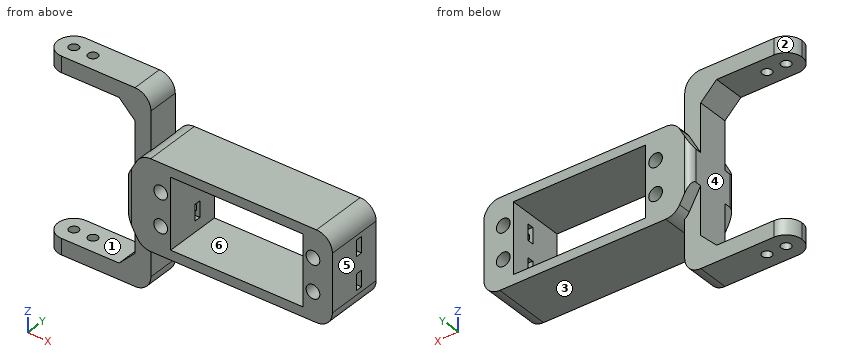
```python
from build123d import *

# Parameters (mm, degrees)
ESQUISSE1_W                         = 60
ESQUISSE1_H                         = 18
BOSS_EXTRU_1_DEPTH                  = 28
ESQUISSE2_W                         = 41.5
ESQUISSE2_H                         = 22
ENL_V_MAT_EXTRU_1_DEPTH             = 30
ESQUISSE3_R                         = 2.15
ENL_V_MAT_EXTRU_2_DEPTH             = 30
ESQUISSE5_W                         = 10
ESQUISSE5_H                         = 60
BOSS_EXTRU_2_DEPTH                  = 5
ESQUISSE6_W                         = 10
ESQUISSE6_H                         = 5
BOSS_EXTRU_3_DEPTH                  = 28
ESQUISSE7_R                         = 1.5
ENL_V_MAT_EXTRU_4_DEPTH             = 92.394748208
NERVURE11_REACH                     = 77.186
ESQUISSE8_WALL_W                    = 162.668500034
ESQUISSE8_WALL_H                    = 18
CONG_5_R                            = 5
CONG_6_R                            = 5
NERVURE12_REACH                     = 73.169
ESQUISSE10_WALL_W                   = 151.408694602
ESQUISSE10_WALL_H                   = 10
CONG_7_R                            = 5
ESQUISSE12_W                        = 5
ESQUISSE12_H                        = 2
ENL_V_MAT_EXTRU_5_DEPTH             = 8
ENL_V_MAT_EXTRU_5_DIRECTION_2_REACH = 67.265
R_P_TITION_CIRCULAIRE1_COUNT        = 3
R_P_TITION_CIRCULAIRE1_ANGLE        = 180
ENL_V_MAT_EXTRU_8_DEPTH             = 79.064076245
ENL_V_MAT_EXTRU_8_DEPTH_BACK        = 79.064076245
CONG_8_R                            = 5
CONG_10_R                           = 5
CONG_12_R                           = 2
NERVURE13_REACH                     = 79.369
ESQUISSE22_WALL_W                   = 163.809556882
ESQUISSE22_WALL_H                   = 10
ENL_V_MAT_EXTRU_10_DEPTH            = 88.464278423
ENL_V_MAT_EXTRU_10_DEPTH_BACK       = 88.464278423
ESQUISSE24_R                        = 1.5


with BuildPart() as part:
    # Esquisse1 → Boss.-Extru.1 (new body)
    with BuildSketch(Plane.XY):
        Rectangle(ESQUISSE1_W, ESQUISSE1_H)
    extrude(amount=BOSS_EXTRU_1_DEPTH)

    # Esquisse2 → Enlèv. mat.-Extru.1 (cut)
    with BuildSketch(Plane.XZ.offset(9)):
        with Locations((0, 14)):
            Rectangle(ESQUISSE2_W, ESQUISSE2_H)
    extrude(amount=-ENL_V_MAT_EXTRU_1_DEPTH, mode=Mode.SUBTRACT)

    # Esquisse3 → Enlèv. mat.-Extru.2 (cut)
    with BuildSketch(Plane(origin=(0, -9, 0), x_dir=(-1, 0, 0), z_dir=(0, -1, 0))):
        with Locations(Location((23.9, -19.1, 0), (0, 0, 90))):
            Circle(ESQUISSE3_R)
        with Locations(Location((23.9, -8.9, 0), (0, 0, 90))):
            Circle(ESQUISSE3_R)
        with Locations(Location((-23.9, -8.9, 0), (0, 0, 90))):
            Circle(ESQUISSE3_R)
        with Locations(Location((-23.9, -19.1, 0), (0, 0, 90))):
            Circle(ESQUISSE3_R)
    extrude(amount=-ENL_V_MAT_EXTRU_2_DEPTH, mode=Mode.SUBTRACT)

    # Esquisse5 → Boss.-Extru.2 (add)
    with BuildSketch(Plane.ZY.offset(30)):
        with Locations((14, 0)):
            Rectangle(ESQUISSE5_W, ESQUISSE5_H)
    boss_extru_2 = extrude(amount=BOSS_EXTRU_2_DEPTH)

    # Esquisse6 → Boss.-Extru.3 (add)
    with BuildSketch(Plane.ZY.offset(35)):
        with Locations((14, 27.5)):
            Rectangle(ESQUISSE6_W, ESQUISSE6_H)
        with Locations((14, -27.5)):
            Rectangle(ESQUISSE6_W, ESQUISSE6_H)
    boss_extru_3 = extrude(amount=BOSS_EXTRU_3_DEPTH)

    # Esquisse7 → Enlèv. mat.-Extru.4 (cut, symmetric)
    with BuildSketch(Plane(origin=(0, 30, 0), x_dir=(1, 0, 0), z_dir=(0, 1, 0))):
        with Locations(Location((-58, -14, 0), (0, 0, 270))):
            Circle(ESQUISSE7_R)
    enl_v_mat_extru_4 = extrude(amount=ENL_V_MAT_EXTRU_4_DEPTH, both=True, mode=Mode.SUBTRACT)

    # Esquisse8 wall → Nervure11 (add, up to next)
    with BuildSketch(Plane(origin=(-32.5, 0, 23.5), x_dir=(-0.485642931179, 0, -0.874157276122), z_dir=(-0.874157276122, 0, 0.485642931179)), mode=Mode.PRIVATE) as nervure11_sk1:
        Rectangle(ESQUISSE8_WALL_W, ESQUISSE8_WALL_H)
    nervure11_tool1 = extrude(nervure11_sk1.sketch, amount=-NERVURE11_REACH, mode=Mode.PRIVATE) - part.part
    nervure11 = nervure11_tool1.solids().sort_by_distance((-32.5, 0, 23.5))[0]
    add(nervure11)

    # Symétrie1: Nervure11 across plane
    add(nervure11.mirror(Plane.XY.offset(14)))

    # Congé5
    cong_5_edges = [part.edges().sort_by_distance(p)[0] for p in [
        (-30, 0, 28),
        (30, 0, 28),
        (-30, 0, 0),
        (30, 0, 0),
    ]]
    fillet(cong_5_edges, radius=CONG_5_R)

    # Congé6
    cong_6_edges = [part.edges().sort_by_distance(p)[0] for p in [
        (-30, 30, 14),
        (-30, -30, 14),
    ]]
    fillet(cong_6_edges, radius=CONG_6_R)

    # Esquisse10 wall → Nervure12 (add, up to next)
    with BuildSketch(Plane(origin=(-37.5, 22.5, 14), x_dir=(0.707106781187, -0.707106781187, 0), z_dir=(0.707106781187, 0.707106781187, 0)), mode=Mode.PRIVATE) as nervure12_sk1:
        Rectangle(ESQUISSE10_WALL_W, ESQUISSE10_WALL_H)
    nervure12_tool1 = extrude(nervure12_sk1.sketch, amount=NERVURE12_REACH, mode=Mode.PRIVATE) - part.part
    nervure12 = nervure12_tool1.solids().sort_by_distance((-37.5, 22.5, 14))[0]
    add(nervure12)

    # Symétrie2: Nervure12 across plane
    add(nervure12.mirror(Plane.ZX))

    # Congé7
    cong_7_edges = [part.edges().sort_by_distance(p)[0] for p in [
        (-63, -27.5, 9),
        (-63, -27.5, 19),
        (-63, 27.5, 9),
        (-63, 27.5, 19),
    ]]
    fillet(cong_7_edges, radius=CONG_7_R - 0.0001)  # a hair under: the kernel refuses the full size

    # Esquisse12 → Enlèv. mat.-Extru.5 (cut)
    with BuildSketch(Plane(origin=(-20.75, 0, 0), x_dir=(0, 0, -1), z_dir=(1, 0, 0))):
        with Locations((-19.1, 2)):
            Rectangle(ESQUISSE12_W, ESQUISSE12_H)
        with Locations((-8.9, 2)):
            Rectangle(ESQUISSE12_W, ESQUISSE12_H)
    extrude(amount=-ENL_V_MAT_EXTRU_5_DEPTH, mode=Mode.SUBTRACT)

    # Esquisse12 → Enlèv. mat.-Extru.5 direction 2 (cut, up to next)
    with BuildSketch(Plane(origin=(-20.75, 0, 0), x_dir=(0, 0, -1), z_dir=(1, 0, 0)), mode=Mode.PRIVATE) as enl_v_mat_extru_5_direction_2_sk1:
        with Locations((-19.1, 2)):
            Rectangle(ESQUISSE12_W, ESQUISSE12_H)
    enl_v_mat_extru_5_direction_2_tool1 = extrude(enl_v_mat_extru_5_direction_2_sk1.sketch, amount=ENL_V_MAT_EXTRU_5_DIRECTION_2_REACH, mode=Mode.PRIVATE) & part.part
    # Esquisse12 → Enlèv. mat.-Extru.5 direction 2 (cut, up to next)
    with BuildSketch(Plane(origin=(-20.75, 0, 0), x_dir=(0, 0, -1), z_dir=(1, 0, 0)), mode=Mode.PRIVATE) as enl_v_mat_extru_5_direction_2_sk2:
        with Locations((-8.9, 2)):
            Rectangle(ESQUISSE12_W, ESQUISSE12_H)
    enl_v_mat_extru_5_direction_2_tool2 = extrude(enl_v_mat_extru_5_direction_2_sk2.sketch, amount=ENL_V_MAT_EXTRU_5_DIRECTION_2_REACH, mode=Mode.PRIVATE) & part.part
    add(enl_v_mat_extru_5_direction_2_tool1.solids().sort_by_distance((-20.75, 2, 19.1))[0], mode=Mode.SUBTRACT)
    add(enl_v_mat_extru_5_direction_2_tool2.solids().sort_by_distance((-20.75, 2, 8.9))[0], mode=Mode.SUBTRACT)

    # Répétition circulaire1: Boss.-Extru.2, Boss.-Extru.3, Enlèv. mat.-Extru.4 ×3 about axis
    r_p_tition_circulaire1_axis = Axis((-35, 0, 14), (-1, 0, 0))
    add([boss_extru_2.rotate(r_p_tition_circulaire1_axis, i * R_P_TITION_CIRCULAIRE1_ANGLE / (R_P_TITION_CIRCULAIRE1_COUNT - 1)) for i in range(1, R_P_TITION_CIRCULAIRE1_COUNT)])
    add([boss_extru_3.rotate(r_p_tition_circulaire1_axis, i * R_P_TITION_CIRCULAIRE1_ANGLE / (R_P_TITION_CIRCULAIRE1_COUNT - 1)) for i in range(1, R_P_TITION_CIRCULAIRE1_COUNT)])
    add([enl_v_mat_extru_4.rotate(r_p_tition_circulaire1_axis, i * R_P_TITION_CIRCULAIRE1_ANGLE / (R_P_TITION_CIRCULAIRE1_COUNT - 1)) for i in range(1, R_P_TITION_CIRCULAIRE1_COUNT)], mode=Mode.SUBTRACT)

    # Esquisse21 → Enlèv. mat.-Extru.8 (cut, two sides: drawn at the far end of the back side and taken through both)
    with BuildSketch(Plane(origin=(0, 0, 9), x_dir=(-1, 0, 0), z_dir=(0, 0, -1)).offset(-ENL_V_MAT_EXTRU_8_DEPTH_BACK)):
        Polygon((63, -25), (40, -25), (35, -20), (35, -9), (30, -9), (30, -30), (63, -30), align=None)
        Polygon((35, 20), (40, 25), (63, 25), (63, 30), (30, 30), (30, 9), (35, 9), align=None)
    extrude(amount=ENL_V_MAT_EXTRU_8_DEPTH + ENL_V_MAT_EXTRU_8_DEPTH_BACK, mode=Mode.SUBTRACT)

    # Congé8
    cong_8_edges = [part.edges().sort_by_distance(p)[0] for p in [
        (-30, 0, 44),
        (-30, 0, -16),
    ]]
    fillet(cong_8_edges, radius=CONG_8_R)

    # Congé10
    cong_10_edges = [part.edges().sort_by_distance(p)[0] for p in [
        (-63, 5, -13.5),
        (-63, -5, -13.5),
        (-63, -5, 41.5),
        (-63, 5, 41.5),
    ]]
    fillet(cong_10_edges, radius=CONG_10_R - 0.0001)  # a hair under: the kernel refuses the full size

    # Congé12
    cong_12_edges = [part.edges().sort_by_distance(p)[0] for p in [
        (-35, -9, 14),
        (-35, 9, 14),
    ]]
    fillet(cong_12_edges, radius=CONG_12_R)

    # Esquisse22 wall → Nervure13 (add, up to next)
    with BuildSketch(Plane(origin=(-37.5, 0, -8.5), x_dir=(0.707106781187, 0, 0.707106781187), z_dir=(0.707106781187, 0, -0.707106781187)), mode=Mode.PRIVATE) as nervure13_sk1:
        Rectangle(ESQUISSE22_WALL_W, ESQUISSE22_WALL_H)
    nervure13_tool1 = extrude(nervure13_sk1.sketch, amount=NERVURE13_REACH, mode=Mode.PRIVATE) - part.part
    nervure13 = nervure13_tool1.solids().sort_by_distance((-37.5, 0, -8.5))[0]
    add(nervure13)

    # Symétrie3: Nervure13 across plane
    add(nervure13.mirror(Plane(origin=(0, 0, 14), x_dir=(1, 0, 0), z_dir=(0, 0, -1))))

    # Esquisse24 → Enlèv. mat.-Extru.10 (cut, two sides: drawn at the far end of the back side and taken through both)
    with BuildSketch(Plane(origin=(0, 0, -16), x_dir=(-1, 0, 0), z_dir=(0, 0, -1)).offset(-ENL_V_MAT_EXTRU_10_DEPTH_BACK)):
        with Locations(Location((52, 0, 0), (0, 0, 90))):
            Circle(ESQUISSE24_R)
    extrude(amount=ENL_V_MAT_EXTRU_10_DEPTH + ENL_V_MAT_EXTRU_10_DEPTH_BACK, mode=Mode.SUBTRACT)


solid = part.part
```
For this review, take the finished solid that the model builds, in its own axes (mm). Face numbers are marked on the shaded views. A direction names the side the tool comes from. Coordinates: 2 decimals unless noted, no trailing zeros. Order: outer loops, then holes, each group sorted by start corner. A loop starts at its lowest first (then second) coordinate and runs counter-clockwise, first axis right, second up. Notation, with made-up numbers: (-27.75, 15.5) -> (-6.75, 15.5) arc R12 ccw to (-6.75, 25.5) -> close; hole circle Ø11 at (39.25, -11). An arc over 180 degrees is marked (long way). Use CSV: the item, a comma, the result in double quotes. Start each with the question number.
Item 1: For the marked faces 4, 5 and 6, list the 3-axis set-ups (+Z, -Z, +X, -X, +Y, -Y) from which the entire face can be reached by the end or side of a thin tool; tool diameter is ignored.
Item 2: We need section B-B, the plane x = 23.9. Give the boundary of the cut face in (y, z), then the cut area to 3 significant figures.
Item 3: We need section C-C, the plane y = -6. Give the boundary of the cut face in (x, z), then the cut area to 3 significant figures.
Item 4: Draft analysis for pull direction Z (two halves, no side actions). For the marked faces 1, 2 and 3, state which applies: pulls with the +Z half, pulls with the -Z half, needs draft (parallel to the pull), parting line crosses it, or undercut.
Item 5: Insertion check: pin 1 (2.5 mm diameter, centred on x = -23.5, z = 8, fed in from -Y); pin 2 (3 mm diameter, centred on x = -18, y = 0, fed in from +Z); pin 3 (10 mm diameter, centred on x = -40.5, z = -2, fed in from +Y); pin 4 (1 mm diameter, centred on y = 2, z = 9.5, fed in from +X). Each pin has a flat end and moves straight along its axis. Give the tip position at first contact, or say it passes through.
Item 6: Wall thickness on probe 1 along Z at (x, y) = (2, 4); probe 2 along X at (y, z) = (5.45, 19.1); probe 3 along Z at (x, y) = (-42.5, 3): over which ranges is each line inside the solid? List them lowest first.
Item 7: We need section D-D, the plane x = -52. Give the boundary of the cut face in (y, z), then the cut area to 3 significant figures.
Item 8: We need section A-A, the plane z = 13.5. Give the boundary of the cut face in (x, y).
Derived:
1,face 4,"-X, +Y, -Y"
1,face 5,"+Z, -Z, +X, +Y, -Y"
1,face 6,"+Y, -Y"
2,outline,"(-9, 0) -> (9, 0) -> (9, 6.75) -> (3, 6.75) -> (3, 6.4) -> (1, 6.4) -> (1, 6.75) -> (-9, 6.75) -> close; (-9, 11.05) -> (1, 11.05) -> (1, 11.4) -> (3, 11.4) -> (3, 11.05) -> (9, 11.05) -> (9, 16.95) -> (3, 16.95) -> (3, 16.6) -> (1, 16.6) -> (1, 16.95) -> (-9, 16.95) -> close; (-9, 21.25) -> (1, 21.25) -> (1, 21.6) -> (3, 21.6) -> (3, 21.25) -> (9, 21.25) -> (9, 28) -> (-9, 28) -> close"
2,area,"346 mm^2"
3,outline,"(-35, 9) -> (-31.43, 2.57) arc R5 ccw to (-27.06, 0) -> (25, 0) arc R5 ccw to (30, 5) -> (30, 23) arc R5 ccw to (25, 28) -> (-27.06, 28) arc R5 ccw to (-31.43, 25.43) -> (-35, 19) -> close; hole circle Ø4.3 at (-23.9, 8.9); hole circle Ø4.3 at (-23.9, 19.1); hole (-20.75, 3) -> (20.75, 3) -> (20.75, 25) -> (-20.75, 25) -> close; hole circle Ø4.3 at (23.9, 8.9); hole circle Ø4.3 at (23.9, 19.1)"
3,area,"790 mm^2"
4,face 1,"undercut"
4,face 2,"needs draft"
4,face 3,"pulls with the -Z half"
5,pin 1,"stops at y = -9"
5,pin 2,"stops at z = 28"
5,pin 3,"passes through"
5,pin 4,"stops at x = -28.75"
6,probe 1,"z = 0 to 3, 25 to 28"
6,probe 2,"x = -34.94 to -26.05, -21.75 to -20.75, 20.75 to 21.75, 26.05 to 30"
6,probe 3,"z = -16 to -11, 39 to 44"
7,outline,"(-5, -16) -> (-1.5, -16) -> (-1.5, -11) -> (-5, -11) -> close; (-5, 39) -> (-1.5, 39) -> (-1.5, 44) -> (-5, 44) -> close; (1.5, -16) -> (5, -16) -> (5, -11) -> (1.5, -11) -> close; (1.5, 39) -> (5, 39) -> (5, 44) -> (1.5, 44) -> close"
7,area,"70.0 mm^2"
8,outline,"(-35, -7) arc R2 ccw to (-33, -9) -> (-20.75, -9) -> (-20.75, 9) -> (-33, 9) arc R2 ccw to (-35, 7) -> close; (20.75, -9) -> (30, -9) -> (30, 9) -> (20.75, 9) -> close"
